Design review of the part built by this model. Coordinates are the model's own, in mm. Face numbers are marked on the shaded views. A direction names the side the tool comes from. Coordinates: 2 decimals unless noted, no trailing zeros. Loops run counter-clockwise (first coordinate to the right, second up) from the corner with the lowest first, then second, coordinate; pieces in that order, holes last. Notation, with made-up numbers: (83, 83.25) - (136, 83.25) arc R21 cw to (136, 108.25) - close; hole circle Ø3 at (53, -8). An arc over 180 degrees is marked (long way). Answer in a Markdown table with one row per item. Add a question column.
(1) The part is to be moulded in two halves that separate along Z. For the marked faces 3, 4, 5 and 6, say which applies: released by +Z, released by -Z, zero draft, split by the parting line, or undercut.
(2) To check wall thickness, follow L1, parallel to X at y = 49, z = 0; L2, parallel to X at y = 14, z = -7.5; L3, parallel to X at y = 21.5, z = -10. State the ranges of each line that lie inside material, in increasing order. Write a range as [from, to].
(3) We need section C-C, the plane y = 55.5. Write out the cut boundary in (x, z), plus the area to 3 significant figures.
(4) We need section D-D, the plane x = -45. Write out the cut boundary in (y, z), plus the area to 3 significant figures.
(5) Clearance check with flat-ended pins moving along their axes: pin 1 (2 mm diameter, centred on x = -1.5, z = -12.5, fed in from -Y); pin 2 (2 mm diameter, centred on x = -37.5, z = 2.5, fed in from +Y); pin 3 (3 mm diameter, centred on y = 25.5, z = -14, fed in from -X); pin 4 (24 mm diameter, centred on x = -38.5, z = -0.5, fed in from +Y). State where each tip first meets the part, or that it passes through.
(6) We need section B-B, the plane x = -80. Write out the cut boundary in (y, z).
(7) We need section A-A, the plane z = 0. Write out the cut boundary in (x, y), plus the area to 3 significant figures.
(8) For the marked faces 1 and 2, list the 3-axis set-ups (+Z, -Z, +X, -X, +Y, -Y) from which the entire face can be reached by the end or side of a thin tool; tool diameter is ignored.
from build123d import *

# Parameters (mm, degrees)
SKETCH5_R            = 10
SKETCH5_R_2          = 40
SKETCH5_R_3          = 25
SKETCH5_R_4          = 15
BOSS_EXTRUDE11_DEPTH = 20
SKETCH11_R           = 25
SKETCH11_R_2         = 15
BOSS_EXTRUDE12_DEPTH = 60
CHAMFER3_SIZE        = 3
FILLET2_R            = 10
CHAMFER4_SIZE        = 3


with BuildPart() as part:
    # Sketch5 → Boss-Extrude11 (new body)
    # profile 1 of 4: a face of its own
    with BuildSketch(Plane(origin=(0, 0, 0), x_dir=(1, 0, 0), z_dir=(0, 1, 0))):
        with BuildLine():
            ThreePointArc((-10, -38.729833462), (-40, 0), (-10, 38.729833462))
            Line((-10, 38.729833462), (-85, 19.364916731))
            ThreePointArc((-85, 19.364916731), (-100, 0), (-85, -19.364916731))
            Line((-85, -19.364916731), (-10, -38.729833462))
        make_face()
        with Locations(Location((-80, 0, 0), (0, 0, 270))):
            Circle(SKETCH5_R, mode=Mode.SUBTRACT)
    # profile 2 of 4: a face of its own
    with BuildSketch(Plane(origin=(0, 0, 0), x_dir=(1, 0, 0), z_dir=(0, 1, 0))):
        with BuildLine():
            Line((85, 19.364916731), (10, 38.729833462))
            ThreePointArc((10, 38.729833462), (31.622776602, 24.494897428), (40, 0))
            ThreePointArc((40, 0), (31.622776602, -24.494897428), (10, -38.729833462))
            Line((10, -38.729833462), (85, -19.364916731))
            ThreePointArc((85, -19.364916731), (100, 0), (85, 19.364916731))
        make_face()
        with Locations(Location((80, 0, 0), (0, 0, 270))):
            Circle(SKETCH5_R, mode=Mode.SUBTRACT)
    # profile 3 of 4: a face of its own
    with BuildSketch(Plane(origin=(0, 0, 0), x_dir=(1, 0, 0), z_dir=(0, 1, 0))):
        Circle(SKETCH5_R_2)
        Circle(SKETCH5_R_3, mode=Mode.SUBTRACT)
    # profile 4 of 4: a face of its own
    with BuildSketch(Plane(origin=(0, 0, 0), x_dir=(1, 0, 0), z_dir=(0, 1, 0))):
        Circle(SKETCH5_R_3)
        with Locations(Location((0, 0, 0), (0, 0, 270))):
            Circle(SKETCH5_R_4, mode=Mode.SUBTRACT)
    extrude(amount=BOSS_EXTRUDE11_DEPTH)

    # Sketch11 → Boss-Extrude12 (add)
    with BuildSketch(Plane.XZ):
        with Locations(Location((0, 0, 0), (0, 0, 270))):
            Circle(SKETCH11_R)
        with Locations(Location((0, 0, 0), (0, 0, 270))):
            Circle(SKETCH11_R_2, mode=Mode.SUBTRACT)
    extrude(amount=-BOSS_EXTRUDE12_DEPTH)

    # Chamfer3
    chamfer3_edges = [part.edges().sort_by_distance(p)[0] for p in [
        (-80, 20, -10),
    ]]
    chamfer(chamfer3_edges, length=CHAMFER3_SIZE)

    # Fillet2
    fillet2_edges = [part.edges().sort_by_distance(p)[0] for p in [
        (0, 20, 25),
    ]]
    fillet(fillet2_edges, radius=FILLET2_R)

    # Chamfer4
    chamfer4_edges = [part.edges().sort_by_distance(p)[0] for p in [
        (80, 20, -10),
    ]]
    chamfer(chamfer4_edges, length=CHAMFER4_SIZE)


solid = part.part
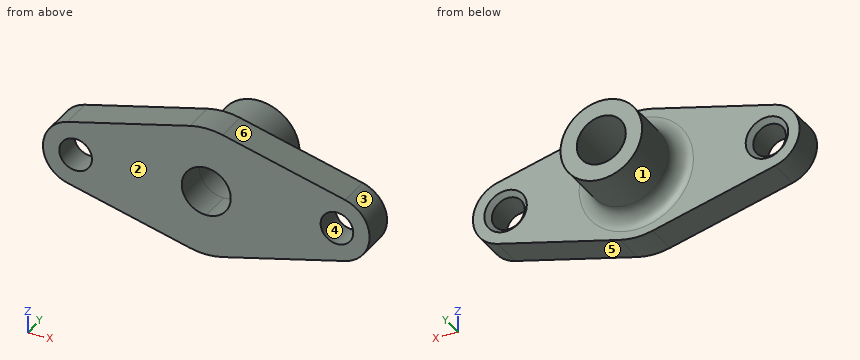
Responses:
| question | item | result |
|---|---|---|
| 1 | face 3 | split by the parting line |
| 1 | face 4 | undercut |
| 1 | face 5 | released by -Z |
| 1 | face 6 | released by +Z |
| 2 | L1 | x = [-25, -15], [15, 25] |
| 2 | L2 | x = [-98.54, -86.61], [-73.39, -12.99], [12.99, 73.39], [86.61, 98.54] |
| 2 | L3 | x = [-28, -11.18], [11.18, 28] |
| 3 | outline | circle Ø50 at (0, 0); hole circle Ø30 at (0, 0) |
| 3 | area | 1,260 mm2 |
| 4 | outline | (0, -29.69) - (20, -29.69) - (20, 29.69) - (0, 29.69) - close |
| 4 | area | 1,190 mm2 |
| 5 | pin 1 | passes through |
| 5 | pin 2 | stops at y = 20 |
| 5 | pin 3 | stops at x = -23.36 |
| 5 | pin 4 | stops at y = 24.73 |
| 6 | outline | (0, -20.66) - (20, -20.66) - (20, -13) - (17, -10) - (0, -10) - close; (0, 10) - (17, 10) - (20, 13) - (20, 20.66) - (0, 20.66) - close |
| 7 | outline | (-100, 0) - (-90, 0) - (-90, 17) - (-93, 20) - (-100, 20) - close; (-70, 0) - (-15, 0) - (-15, 60) - (-25, 60) - (-25, 30) arc R10 cw to (-35, 20) - (-67, 20) - (-70, 17) - close; (15, 0) - (70, 0) - (70, 17) - (67, 20) - (35, 20) arc R10 cw to (25, 30) - (25, 60) - (15, 60) - close; (90, 0) - (100, 0) - (100, 20) - (93, 20) - (90, 17) - close |
| 7 | area | 3,420 mm2 |
| 8 | face 1 | +Y |
| 8 | face 2 | +Z, -Z, +X, -X, -Y |
